```python
from build123d import *

# Parameters (mm, degrees)
SKETCH1_W                = 70
SKETCH1_H                = 150
BOSS_EXTRUDE1_DEPTH      = 5
SKETCH2_W                = 3
SKETCH2_H                = 15
BOSS_EXTRUDE3_DEPTH      = 20
SKETCH2_5_W              = 16
SKETCH2_5_H              = 22
SKETCH2_5_W_2            = 3
SKETCH2_5_H_2            = 15
BOSS_EXTRUDE4_DEPTH      = 5
CHAMFER1_SIZE            = 3
SKETCH3_R                = 3
CUT_EXTRUDE1_DEPTH       = 89.600225733
CHAMFER3_SIZE            = 1
CHAMFER4_SIZE            = 1
CHAMFER5_SIZE            = 3
CHAMFER6_SIZE            = 3
CHAMFER7_SIZE            = 20
CHAMFER8_SIZE            = 10
SKETCH4_W                = 3
SKETCH4_H                = 10
BOSS_EXTRUDE5_DEPTH      = 10
SKETCH6_R                = 1.5
CUT_EXTRUDE2_DEPTH       = 88.076116128
FILLET1_R                = 5
CHAMFER10_SIZE           = 1
CUT_EXTRUDE3_DEPTH       = 87
BOSS_EXTRUDE6_DEPTH      = 5
BOSS_EXTRUDE6_DEPTH_BACK = 7.5
SKETCH8_W                = 18
SKETCH8_H                = 2
FILLET2_R                = 2
FILLET3_R                = 1


# Some blends are built 0.0001 mm under size
with BuildPart() as part:
    # Sketch1 → Boss-Extrude1 (new body)
    with BuildSketch(Plane(origin=(0, 0, 0), x_dir=(1, 0, 0), z_dir=(0, 1, 0))):
        Rectangle(SKETCH1_W, SKETCH1_H)
    extrude(amount=BOSS_EXTRUDE1_DEPTH)

    # Sketch2 → Boss-Extrude3 (add)
    with BuildSketch(Plane(origin=(0, 5, 0), x_dir=(1, 0, 0), z_dir=(0, 1, 0))):
        with Locations((3.5, 62.5)):
            Rectangle(SKETCH2_W, SKETCH2_H)
        with Locations((-3.5, 62.5)):
            Rectangle(SKETCH2_W, SKETCH2_H)
    extrude(amount=BOSS_EXTRUDE3_DEPTH)

    # Sketch2<5> → Boss-Extrude4 (add)
    with BuildSketch(Plane(origin=(0, 5, 0), x_dir=(1, 0, 0), z_dir=(0, 1, 0))):
        with Locations((0, 62.5)):
            Rectangle(SKETCH2_5_W, SKETCH2_5_H)
        with Locations((-3.5, 62.5)):
            Rectangle(SKETCH2_5_W_2, SKETCH2_5_H_2, mode=Mode.SUBTRACT)
        with Locations((3.5, 62.5)):
            Rectangle(SKETCH2_5_W_2, SKETCH2_5_H_2, mode=Mode.SUBTRACT)
    extrude(amount=BOSS_EXTRUDE4_DEPTH)

    # Chamfer1
    chamfer1_edges = [part.edges().sort_by_distance(p)[0] for p in [
        (0, 10, -73.5),
        (0, 10, -51.5),
    ]]
    chamfer(chamfer1_edges, length=CHAMFER1_SIZE)

    # Sketch3 → Cut-Extrude1 (cut, through all)
    with BuildSketch(Plane(origin=(5, 0, 0), x_dir=(0, 0, -1), z_dir=(1, 0, 0))):
        with Locations((62.5, 23.2)):
            Circle(SKETCH3_R)
    extrude(amount=-CUT_EXTRUDE1_DEPTH, mode=Mode.SUBTRACT)

    # Chamfer3
    # the kernel refuses this chamfer: 1, 0.714285714 mm, written as the material it takes off along each edge
    with BuildSketch(Plane(origin=(-7.571682988, 25, -64.9), x_dir=(0, -0.8672694366120031, -0.4978390546338231), z_dir=(1, 0, 0)), Plane(origin=(-0.571682988, 25, -64.9), x_dir=(0, -0.8672694366120031, -0.4978390546338231), z_dir=(1, 0, 0))) as chamfer3_piece_1:
        with BuildLine():
            Line((0.73254251, 0), (CHAMFER3_SIZE * 0.497839054634, CHAMFER3_SIZE * 0.867269436612))
            Line((CHAMFER3_SIZE * 0.497839054634, CHAMFER3_SIZE * 0.867269436612), (0, 0))
            ThreePointArc((0, 0), (0.371569513, 0.022438375), (0.73254251, 0))
        make_face()
    extrude(amount=8.143365976, mode=Mode.SUBTRACT)
    with BuildSketch(Plane(origin=(-7.571682988, 25, -60.1), x_dir=(0, 0, 1), z_dir=(1, 0, 0)), Plane(origin=(-0.571682988, 25, -60.1), x_dir=(0, 0, 1), z_dir=(1, 0, 0))) as chamfer3_piece_2:
        with BuildLine():
            Line((CHAMFER3_SIZE, 0), (0.36468827, 0.63531173))
            ThreePointArc((0.36468827, 0.63531173), (0.204441932, 0.311080183), (0, 0))
            Line((0, 0), (CHAMFER3_SIZE, 0))
        make_face()
    extrude(amount=8.143365976, mode=Mode.SUBTRACT)

    # Chamfer4
    chamfer4_edges = [part.edges().sort_by_distance(p)[0] for p in [
        (3.5, 25, -70),
        (3.5, 25, -55),
        (-3.5, 25, -70),
        (-3.5, 25, -55),
    ]]
    chamfer(chamfer4_edges, length=CHAMFER4_SIZE)

    # Chamfer5
    # the kernel refuses this chamfer: 3 mm, written as the material it adds along each edge
    with BuildSketch(Plane(origin=(-8, 5, -73.5), x_dir=(0, 1, 0), z_dir=(0, 0, 1))) as chamfer5_piece_1_section:
        Polygon((CHAMFER5_SIZE, 0), (0, CHAMFER5_SIZE), (0, 0), align=None)
    chamfer5_piece_1 = extrude(amount=22, mode=Mode.PRIVATE)
    chamfer5_piece_1 = split(chamfer5_piece_1, bisect_by=Plane(origin=(-8, 17, -61.5), z_dir=(0, -0.7071067811865476, -0.7071067811865476)), keep=Keep.TOP, mode=Mode.PRIVATE)
    chamfer5_piece_1 = split(chamfer5_piece_1, bisect_by=Plane(origin=(-8, 6, -74.5), z_dir=(0, -0.7071067811865476, 0.7071067811865476)), keep=Keep.TOP, mode=Mode.PRIVATE)
    add(chamfer5_piece_1)
    with BuildSketch(Plane(origin=(8, 5, -51.5), x_dir=(0, 1, 0), z_dir=(0, 0, -1))) as chamfer5_piece_2_section:
        Polygon((CHAMFER5_SIZE, 0), (0, CHAMFER5_SIZE), (0, 0), align=None)
    chamfer5_piece_2 = extrude(amount=22, mode=Mode.PRIVATE)
    chamfer5_piece_2 = split(chamfer5_piece_2, bisect_by=Plane(origin=(8, 6, -50.5), z_dir=(0, -0.7071067811865476, -0.7071067811865476)), keep=Keep.TOP, mode=Mode.PRIVATE)
    chamfer5_piece_2 = split(chamfer5_piece_2, bisect_by=Plane(origin=(8, 17, -63.5), z_dir=(0, -0.7071067811865476, 0.7071067811865476)), keep=Keep.TOP, mode=Mode.PRIVATE)
    add(chamfer5_piece_2)

    # Chamfer6
    chamfer6_edges = [part.edges().sort_by_distance(p)[0] for p in [
        (-5, 10, -62.5),
        (5, 10, -62.5),
    ]]
    chamfer(chamfer6_edges, length=CHAMFER6_SIZE - 0.0001)  # a hair under: the kernel refuses the full size

    # Chamfer7
    chamfer7_edges = [part.edges().sort_by_distance(p)[0] for p in [
        (35, 2.5, 75),
        (-35, 2.5, 75),
    ]]
    chamfer(chamfer7_edges, length=CHAMFER7_SIZE)

    # Chamfer8
    chamfer8_edges = [part.edges().sort_by_distance(p)[0] for p in [
        (-35, 2.5, -75),
        (35, 2.5, -75),
    ]]
    chamfer(chamfer8_edges, length=CHAMFER8_SIZE)

    # Sketch4 → Boss-Extrude5 (add)
    with BuildSketch(Plane(origin=(0, 5, 0), x_dir=(1, 0, 0), z_dir=(0, 1, 0))):
        with Locations((0, -70)):
            Rectangle(SKETCH4_W, SKETCH4_H)
    extrude(amount=BOSS_EXTRUDE5_DEPTH)

    # Sketch6 → Cut-Extrude2 (cut, through all)
    with BuildSketch(Plane(origin=(1.5, 0, 0), x_dir=(0, 0, -1), z_dir=(1, 0, 0))):
        with Locations((-70, 12)):
            Circle(SKETCH6_R)
    extrude(amount=-CUT_EXTRUDE2_DEPTH, mode=Mode.SUBTRACT)

    # Fillet1
    fillet1_edges = [part.edges().sort_by_distance(p)[0] for p in [
        (0, 15, 75),
        (0, 15, 65),
    ]]
    fillet(fillet1_edges, radius=FILLET1_R - 0.0001)  # a hair under: the kernel refuses the full size

    # Chamfer10
    chamfer10_edges = [part.edges().sort_by_distance(p)[0] for p in [
        (0, 0, 75),
        (35, 0, -5),
        (25, 0, 65),
        (-25, 0, 65),
        (-35, 0, -5),
        (0, 0, -75),
        (30, 0, -70),
        (-30, 0, -70),
    ]]
    chamfer(chamfer10_edges, length=CHAMFER10_SIZE)

    # Sketch7 → Cut-Extrude3 (cut)
    with BuildSketch(Plane.ZY.offset(35)):
        Polygon((-104.766483953, 57.568464944), (-5.977667253, 57.568464944), (-5.977667253, 5), (81.485043075, 5), (81.485043075, -30.208859449), (-5.977667253, -30.208859449), (-5.977667253, -7.084725604), (-104.766483953, -7.084725604), align=None)
    extrude(amount=-CUT_EXTRUDE3_DEPTH, mode=Mode.SUBTRACT)

    # Sketch8 → Boss-Extrude6 (add, two sides: drawn at the far end of the back side and taken through both)
    with BuildSketch(Plane.ZY.offset(1.5).offset(-BOSS_EXTRUDE6_DEPTH_BACK)):
        with Locations((70, 6)):
            Rectangle(SKETCH8_W, SKETCH8_H)
    extrude(amount=BOSS_EXTRUDE6_DEPTH + BOSS_EXTRUDE6_DEPTH_BACK)

    # Fillet2
    fillet2_edges = [part.edges().sort_by_distance(p)[0] for p in [
        (0, 7, 75),
        (0, 7, 65),
    ]]
    fillet(fillet2_edges, radius=FILLET2_R)

    # Fillet3
    fillet3_edges = [part.edges().sort_by_distance(p)[0] for p in [
        (6, 6, 61),
        (6, 6, 79),
        (-6.5, 6, 61),
        (-6.5, 6, 79),
    ]]
    fillet(fillet3_edges, radius=FILLET3_R)


solid = part.part
```
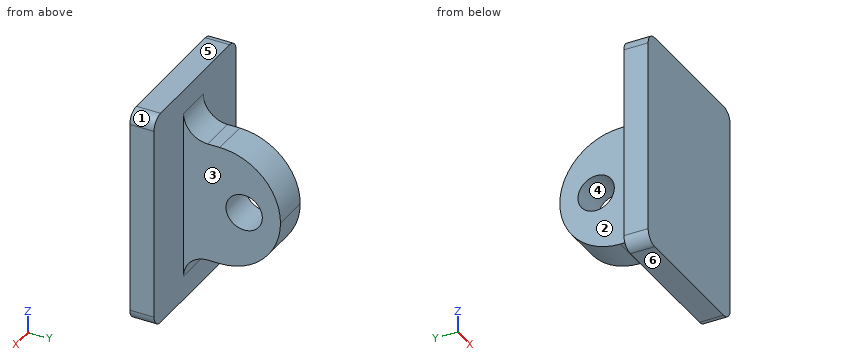
Part model, mm, in its own coordinate system. Face numbers are marked on the shaded views. A direction names the side the tool comes from. Round coordinates to 2 decimals unless told otherwise and drop trailing zeros. Loops run counter-clockwise (first coordinate to the right, second up) from the corner with the lowest first, then second, coordinate; pieces in that order, holes last.
Item 1: Drop flat-ended pins along their axis: P1, Ø1.5, axis at x = 3.5, z = 65, coming from the +Y side; P2, Ø3, axis at y = 13.5, z = 65, coming from the -X side; P3, Ø0.5, axis at x = 0.5, y = 9.5, coming from the -Z side; P4, Ø2, axis at x = 3.5, y = 9.5, coming from the +Z side. Give the stop position or say it passes through.
Item 2: Drill centre lines: line 1 (Y direction, x = 0.2, z = 70); line 2 (X direction, y = 12.25, z = 74.25); line 3 (Y direction, x = 4.25, z = 65). Where is each one in solid material? Low to high.
Item 3: Cut at D-D, the plane z = 64. Give the cut face in (x, y), then the cut area to 3 significant figures.
Item 4: Cut at B-B, the plane y = 12. Give the cut face in (x, z).
Item 5: 3-axis set-ups, long thin cutter, end or side, ignore diameter. For the marked faces 1 and 2: which of +Z, -Z, +X, -X, +Y, -Y reach the whole face in a straight line?
Item 6: Mould opens along Z. For the marked faces 3, 4, 5 and 6 say: +Z half, -Z half, draft (parallel to the pull), parting line (faces both ways), or undercut.
Item 7: Cut at A-A, the plane z = 69.5. Give the cut face in (x, y), then the cut area to 3 significant figures.
A:
1. P1: stops at y = 7
1. P2: stops at x = -1.5
1. P3: stops at z = 65
1. P4: passes through
2. line 1: y = 5 to 10.5, 13.5 to 15
2. line 2: x = -1.5 to 1.5
2. line 3: y = 5 to 7
3. outline: (-6.5, 5) - (6, 5) - (6, 7) - (1.5, 7) - (1.5, 7.27) - (-1.5, 7.27) - (-1.5, 7) - (-6.5, 7) - close
3. area: 25.8 mm2
4. outline: (-1.5, 65.42) - (1.5, 65.42) - (1.5, 68.5) - (-1.5, 68.5) - close; (-1.5, 71.5) - (1.5, 71.5) - (1.5, 74.58) - (-1.5, 74.58) - close
5. face 1: +Z, +X, +Y, -Y
5. face 2: +Z, -Z, -X, +Y
6. face 3: draft
6. face 4: undercut
6. face 5: +Z half
6. face 6: -Z half
7. outline: (-6.5, 5) - (6, 5) - (6, 7) - (1.5, 7) - (1.5, 10.59) - (-1.5, 10.59) - (-1.5, 7) - (-6.5, 7) - close; (-1.5, 13.41) - (1.5, 13.41) - (1.5, 14.97) - (-1.5, 14.97) - close
7. area: 40.4 mm2
